For this review, take the finished solid that the model builds, in its own axes (mm). Face numbers are marked on the shaded views. A direction names the side the tool comes from. Round coordinates to 2 decimals unless told otherwise and drop trailing zeros. Write each loop counter-clockwise with the first axis right and the second up, starting at its lowest first coordinate (ties: lowest second). Pieces come first, ordered by that corner, then holes. Notation, with made-up numbers: (-11, 15) - (41, 15) arc R14 ccw to (41, 19) - close; hole circle Ø1 at (-30, 61). An arc over 180 degrees is marked (long way). One line per item, written item: value. Start each with the question number.
Q1. For probe 1 along X at (y, z) = (-23, 53.25); probe 2 along Y at (x, z) = (-32.5, 56); probe 3 along X at (y, z) = (41, 53), list the stretches that pass through material, from the lowest coordinate up.
Q2. Clearance check with flat-ended pins moving along their axes: pin 1 Ø2.5 at (x, y) = (-38.8, 16.07) entering from -Z; pin 2 Ø1.5 at (x, z) = (26, 44.5) entering from +Y; pin 3 Ø4 at (y, z) = (13, 57) entering from +X; pin 4 Ø10 at (x, z) = (-22, 52) entering from -Y. State where each tip first meets the part, or that it passes through.
Q3. Add section A-A on x = 0. Write out the cut boundary in (y, z).
Q4. Add section D-D on z = 59. Give the number of separate pieces and of enclosed holes in the cut face, and give its area (3 significant figures).
Q5. Mouldability with a two-part tool opening along Y and no side actions: class the marked faces 4, 5 and 6 as +Y half, -Y half, draft (parallel to the pull), parting line (faces both ways), or undercut.
Q6. Add section B-B on y = 4. Write out the cut boundary in (x, z).
Q7. Add section C-C on x = 13. Write out the cut boundary in (y, z), and give its area (3 significant figures).
Q8. Tool access review of the marked faces 1, 2 and 3: name each direction out of +Z, -Z, +X, -X, +Y, -Y from which nothing blocks a thin tool from reaching the whole face with its end or side.
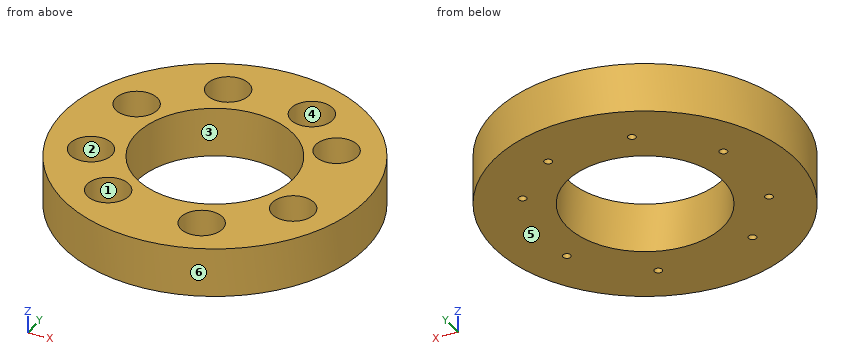
```python
from build123d import *

# Parameters (mm, degrees)
CYLINDER430_R               = 1.5
CYLINDER430_DEPTH           = 100
CYLINDER432_R               = 1.5
CYLINDER432_DEPTH           = 100
CYLINDER432_ROLL_ANGLE      = -0.500355
CYLINDER432_PITCH_ANGLE     = 0.967193
CYLINDER432_PLACEMENT_ANGLE = 144.93646
CYLINDER434_R               = 1.5
CYLINDER434_DEPTH           = 100
CYLINDER436_R               = 1.5
CYLINDER436_DEPTH           = 100
CYLINDER436_PLACEMENT_ANGLE = 225
CYLINDER438_R               = 1.5
CYLINDER438_DEPTH           = 100
CYLINDER440_R               = 1.5
CYLINDER440_DEPTH           = 100
CYLINDER440_PLACEMENT_ANGLE = 45
CYLINDER442_R               = 1.5
CYLINDER442_DEPTH           = 100
CYLINDER442_ROLL_ANGLE      = 0.146073
CYLINDER442_PITCH_ANGLE     = 1.079101
CYLINDER442_PLACEMENT_ANGLE = -9.939308
CYLINDER428_R               = 1.5
CYLINDER428_DEPTH           = 100
CYLINDER428_PLACEMENT_ANGLE = 45
CYLINDER439_R               = 8
CYLINDER439_DEPTH           = 18
CYLINDER437_R               = 8
CYLINDER437_DEPTH           = 18
CYLINDER437_PLACEMENT_ANGLE = 225
CYLINDER435_R               = 8
CYLINDER435_DEPTH           = 18
CYLINDER433_R               = 8
CYLINDER433_DEPTH           = 18
CYLINDER433_ROLL_ANGLE      = -0.500355
CYLINDER433_PITCH_ANGLE     = 0.967193
CYLINDER433_PLACEMENT_ANGLE = 144.93646
CYLINDER431_R               = 8
CYLINDER431_DEPTH           = 18
CYLINDER429_R               = 8
CYLINDER429_DEPTH           = 18
CYLINDER429_PLACEMENT_ANGLE = 45
CYLINDER443_R               = 8
CYLINDER443_DEPTH           = 18
CYLINDER443_ROLL_ANGLE      = 0.146073
CYLINDER443_PITCH_ANGLE     = 1.079101
CYLINDER443_PLACEMENT_ANGLE = -9.939308
CYLINDER441_R               = 8
CYLINDER441_DEPTH           = 18
CYLINDER441_PLACEMENT_ANGLE = 45
TUBE022_R                   = 58
TUBE022_R_2                 = 30
TUBE022_DEPTH               = 19


with BuildPart() as obj1:
    # Cylinder430 → Cylinder430 (new body)
    with BuildSketch(Plane(origin=(38.80294, -16.072704, 0), x_dir=(0, 1, 0), z_dir=(0, 0, 1))):
        Circle(CYLINDER430_R)
    extrude(amount=CYLINDER430_DEPTH)


with BuildPart() as obj2:
    # Cylinder432 → Cylinder432 (new body)
    with BuildSketch(Plane.XY):
        Circle(CYLINDER432_R)
    extrude(amount=CYLINDER432_DEPTH)


with BuildPart() as obj2_1:
    # Cylinder432 roll: moved
    add(obj2.part.rotate(Axis((0, 0, 0), (1, 0, 0)), CYLINDER432_ROLL_ANGLE))


with BuildPart() as obj2_2:
    # Cylinder432 pitch: moved
    add(obj2_1.part.rotate(Axis((0, 0, 0), (0, 1, 0)), CYLINDER432_PITCH_ANGLE))


with BuildPart() as obj2_3:
    # Cylinder432 placement: moved
    add(obj2_2.part.moved(Location((35.440039, 22.530677, 0.610113))).rotate(Axis((35.440039, 22.530677, 0.610113), (0, 0, 1)), CYLINDER432_PLACEMENT_ANGLE))


with BuildPart() as obj3:
    # Cylinder434 → Cylinder434 (new body)
    with BuildSketch(Plane(origin=(16.072704, 38.80294, 0), x_dir=(-1, 0, 0), z_dir=(0, 0, 1))):
        Circle(CYLINDER434_R)
    extrude(amount=CYLINDER434_DEPTH)


with BuildPart() as obj4:
    # Cylinder436 → Cylinder436 (new body)
    with BuildSketch(Plane.XY):
        Circle(CYLINDER436_R)
    extrude(amount=CYLINDER436_DEPTH)


with BuildPart() as obj4_1:
    # Cylinder436 placement: moved
    add(obj4.part.moved(Location((-16.072704, 38.80294, 0))).rotate(Axis((-16.072704, 38.80294, 0), (0, 0, 1)), CYLINDER436_PLACEMENT_ANGLE))


with BuildPart() as obj5:
    # Cylinder438 → Cylinder438 (new body)
    with BuildSketch(Plane(origin=(-38.80294, 16.072704, 0), x_dir=(0, -1, 0), z_dir=(0, 0, 1))):
        Circle(CYLINDER438_R)
    extrude(amount=CYLINDER438_DEPTH)


with BuildPart() as obj6:
    # Cylinder440 → Cylinder440 (new body)
    with BuildSketch(Plane.XY):
        Circle(CYLINDER440_R)
    extrude(amount=CYLINDER440_DEPTH)


with BuildPart() as obj6_1:
    # Cylinder440 placement: moved
    add(obj6.part.moved(Location((-38.80294, -16.072704, 0))).rotate(Axis((-38.80294, -16.072704, 0), (0, 0, -1)), CYLINDER440_PLACEMENT_ANGLE))


with BuildPart() as obj7:
    # Cylinder442 → Cylinder442 (new body)
    with BuildSketch(Plane.XY):
        Circle(CYLINDER442_R)
    extrude(amount=CYLINDER442_DEPTH)


with BuildPart() as obj7_1:
    # Cylinder442 roll: moved
    add(obj7.part.rotate(Axis((0, 0, 0), (1, 0, 0)), CYLINDER442_ROLL_ANGLE))


with BuildPart() as obj7_2:
    # Cylinder442 pitch: moved
    add(obj7_1.part.rotate(Axis((0, 0, 0), (0, 1, 0)), CYLINDER442_PITCH_ANGLE))


with BuildPart() as obj7_3:
    # Cylinder442 placement: moved
    add(obj7_2.part.moved(Location((-22.528054, -35.446371, 0.203785))).rotate(Axis((-22.528054, -35.446371, 0.203785), (0, 0, 1)), CYLINDER442_PLACEMENT_ANGLE))


with BuildPart() as compound321:
    # Cylinder428 → Cylinder428 (new body)
    with BuildSketch(Plane.XY):
        Circle(CYLINDER428_R)
    extrude(amount=CYLINDER428_DEPTH)


with BuildPart() as compound321_1:
    # Cylinder428 placement: moved
    add(compound321.part.moved(Location((16.072704, -38.80294, 0))).rotate(Axis((16.072704, -38.80294, 0), (0, 0, 1)), CYLINDER428_PLACEMENT_ANGLE))

    # Compound321: union obj1, obj2, obj3, obj4, obj5, obj6, obj7
    add(obj1.part)
    add(obj2_3.part)
    add(obj3.part)
    add(obj4_1.part)
    add(obj5.part)
    add(obj6_1.part)
    add(obj7_3.part)


with BuildPart() as obj8:
    # Cylinder439 → Cylinder439 (new body)
    with BuildSketch(Plane(origin=(-38.798949, 16.072537, 43), x_dir=(0, -1, 0), z_dir=(0, 0, 1))):
        Circle(CYLINDER439_R)
    extrude(amount=CYLINDER439_DEPTH)


with BuildPart() as obj9:
    # Cylinder437 → Cylinder437 (new body)
    with BuildSketch(Plane.XY):
        Circle(CYLINDER437_R)
    extrude(amount=CYLINDER437_DEPTH)


with BuildPart() as obj9_1:
    # Cylinder437 placement: moved
    add(obj9.part.moved(Location((-16.07, 38.8, 43))).rotate(Axis((-16.07, 38.8, 43), (0, 0, 1)), CYLINDER437_PLACEMENT_ANGLE))


with BuildPart() as obj10:
    # Cylinder435 → Cylinder435 (new body)
    with BuildSketch(Plane(origin=(16.072537, 38.798949, 43), x_dir=(-1, 0, 0), z_dir=(0, 0, 1))):
        Circle(CYLINDER435_R)
    extrude(amount=CYLINDER435_DEPTH)


with BuildPart() as obj11:
    # Cylinder433 → Cylinder433 (new body)
    with BuildSketch(Plane.XY):
        Circle(CYLINDER433_R)
    extrude(amount=CYLINDER433_DEPTH)


with BuildPart() as obj11_1:
    # Cylinder433 roll: moved
    add(obj11.part.rotate(Axis((0, 0, 0), (1, 0, 0)), CYLINDER433_ROLL_ANGLE))


with BuildPart() as obj11_2:
    # Cylinder433 pitch: moved
    add(obj11_1.part.rotate(Axis((0, 0, 0), (0, 1, 0)), CYLINDER433_PITCH_ANGLE))


with BuildPart() as obj11_3:
    # Cylinder433 placement: moved
    add(obj11_2.part.moved(Location((34.627801, 22.637113, 43.602309))).rotate(Axis((34.627801, 22.637113, 43.602309), (0, 0, 1)), CYLINDER433_PLACEMENT_ANGLE))


with BuildPart() as obj12:
    # Cylinder431 → Cylinder431 (new body)
    with BuildSketch(Plane(origin=(38.798949, -16.072537, 43), x_dir=(0, 1, 0), z_dir=(0, 0, 1))):
        Circle(CYLINDER431_R)
    extrude(amount=CYLINDER431_DEPTH)


with BuildPart() as obj13:
    # Cylinder429 → Cylinder429 (new body)
    with BuildSketch(Plane.XY):
        Circle(CYLINDER429_R)
    extrude(amount=CYLINDER429_DEPTH)


with BuildPart() as obj13_1:
    # Cylinder429 placement: moved
    add(obj13.part.moved(Location((16.07, -38.8, 43))).rotate(Axis((16.07, -38.8, 43), (0, 0, 1)), CYLINDER429_PLACEMENT_ANGLE))


with BuildPart() as obj14:
    # Cylinder443 → Cylinder443 (new body)
    with BuildSketch(Plane.XY):
        Circle(CYLINDER443_R)
    extrude(amount=CYLINDER443_DEPTH)


with BuildPart() as obj14_1:
    # Cylinder443 roll: moved
    add(obj14.part.rotate(Axis((0, 0, 0), (1, 0, 0)), CYLINDER443_ROLL_ANGLE))


with BuildPart() as obj14_2:
    # Cylinder443 pitch: moved
    add(obj14_1.part.rotate(Axis((0, 0, 0), (0, 1, 0)), CYLINDER443_PITCH_ANGLE))


with BuildPart() as obj14_3:
    # Cylinder443 placement: moved
    add(obj14_2.part.moved(Location((-21.748471, -35.690226, 43.196026))).rotate(Axis((-21.748471, -35.690226, 43.196026), (0, 0, 1)), CYLINDER443_PLACEMENT_ANGLE))


with BuildPart() as compound323:
    # Cylinder441 → Cylinder441 (new body)
    with BuildSketch(Plane.XY):
        Circle(CYLINDER441_R)
    extrude(amount=CYLINDER441_DEPTH)


with BuildPart() as compound323_1:
    # Cylinder441 placement: moved
    add(compound323.part.moved(Location((-38.8, -16.07, 43))).rotate(Axis((-38.8, -16.07, 43), (0, 0, -1)), CYLINDER441_PLACEMENT_ANGLE))

    # Compound323: union obj8, obj9, obj10, obj11, obj12, obj13, obj14
    add(obj8.part)
    add(obj9_1.part)
    add(obj10.part)
    add(obj11_3.part)
    add(obj12.part)
    add(obj13_1.part)
    add(obj14_3.part)


with BuildPart() as compound323_2:
    # Compound323 placement: moved
    add(compound323_1.part.moved(Location((0, 0, 3))))


with BuildPart() as obj15:
    # Tube022 → Tube022 (new body)
    with BuildSketch(Plane.XY.offset(42)):
        Circle(TUBE022_R)
        Circle(TUBE022_R_2, mode=Mode.SUBTRACT)
    extrude(amount=TUBE022_DEPTH)

    # Cut169: cut Compound323
    add(compound323_2.part, mode=Mode.SUBTRACT)

    # Cut170: cut Compound321
    add(compound321_1.part, mode=Mode.SUBTRACT)


solid = obj15.part
```
Result set:
1. probe 1: x = -53.24 to -42.8, -34.8 to -19.26, 19.26 to 34.8, 42.8 to 53.24
1. probe 2: y = -48.04 to -21, -11.14 to 11.14, 21 to 48.04
1. probe 3: x = -41.02 to -23.76, -8.38 to 8.38, 23.76 to 41.02
2. pin 1: passes through
2. pin 2: stops at y = 52.22
2. pin 3: stops at x = 56.95
2. pin 4: stops at y = -55.45
3. outline: (-58, 42) - (-30, 42) - (-30, 61) - (-58, 61) - close; (30, 42) - (58, 42) - (58, 61) - (30, 61) - close
4. separate pieces: 1
4. enclosed holes: 9
4. area: 6,130 mm^2
5. face 4: undercut
5. face 5: draft
5. face 6: parting line
6. outline: (-57.86, 42) - (-29.73, 42) - (-29.73, 61) - (-57.86, 61) - close; (29.73, 42) - (57.86, 42) - (57.86, 61) - (29.73, 61) - close
7. outline: (-56.52, 42) - (-27.04, 42) - (-27.04, 61) - (-31.41, 61) - (-31.41, 46) - (-46.19, 46) - (-46.19, 61) - (-56.52, 61) - close; (27.04, 42) - (56.52, 42) - (56.52, 61) - (46.19, 61) - (46.19, 46) - (31.41, 46) - (31.41, 61) - (27.04, 61) - close
7. area: 677 mm^2
8. face 1: none
8. face 2: +Z
8. face 3: +Z, -Z
